Autodesk Inventor part; units mm, degrees
ref_plane "YZ Plane" through (0, 0, 0) normal (1, 0, 0) x (0, 1, 0)
ref_plane "XZ Plane" through (0, 0, 0) normal (0, 1, 0) x (-1, 0, 0)
ref_plane "XY Plane" through (0, 0, 0) normal (0, 0, 1) x (1, 0, 0)
sketch "Sketch1" plane through (0, 0, 0) normal (0, 1, 0) x (-1, 0, 0)
  line L0 (0, 0) -> (37, 0)
  line L1 (37, 0) -> (37, -119)
  line L2 (37, -119) -> (0, -119)
  line L3 (0, -119) -> (0, 0)
  dimension "d0" = 37
  dimension "d1" = 119
extrude "Extrusion1" add sketch "Sketch1" along normal blind 2
sketch "Sketch3" plane through (0, 0, 0) normal (0, -1, 0) x (1, 0, 0)
  line L0 (0, 0) -> (-16.5, 0)
  line L1 (-37, 0) -> (0, 0)
  line L2 (-19, 0) -> (-19, -2)
  arc A0 (-21.5, -2) -> (-16.5, -2) centre (-19, -2) ccw
  line L3 (0, 0) -> (0, -119)
  line L4 (0, -119) -> (-19, -119)
  line L5 (0, -119) -> (-37, -119)
  line L6 (-19, -119) -> (-19, -117)
  arc A1 (-16.5, -117) -> (-21.5, -117) centre (-19, -117) ccw
  line L7 (-16.5, -117) -> (-16.5, -119)
  line L8 (-21.5, -117) -> (-21.5, -119)
  line L9 (-21.5, -119) -> (-16.5, -119)
  line L10 (-21.5, -2) -> (-21.5, 0)
  line L11 (-16.5, -2) -> (-16.5, 0)
  line L12 (-21.5, 0) -> (-16.5, 0)
  dimension "d14" = 19
  dimension "d15" = 2
  dimension "d16" = 5
  dimension "d17" = 19
  dimension "d18" = 2
  dimension "d19" = 5
extrude "Extrusion3" cut sketch "Sketch3" against normal blind 2
sketch "Sketch4" plane through (0, 2, 0) normal (0, 1, 0) x (1, 0, 0)
  line L0 (0, 119) -> (0, 0)
  line L1 (0, 0) -> (0, 12)
  line L2 (0, 12) -> (-6, 12)
  line L3 (-32, 12) -> (-32, 105)
  line L4 (-6, 105) -> (-6, 12)
  line L5 (-11.7, 105) -> (-11.7, 108.4)
  line L6 (-11.7, 108.4) -> (-10.4, 108.4)
  line L7 (-10.4, 108.4) -> (-10.4, 105)
  line L8 (-6, 12) -> (-8, 12)
  line L9 (-8, 12) -> (-8, 105)
  line L10 (-11.7, 105) -> (-11.7, 102)
  line L11 (-11.7, 102) -> (-10.2, 102)
  line L12 (-10.2, 102) -> (-10.2, 15)
  line L13 (-32, 105) -> (-11.7, 105)
  line L14 (-10.2, 15) -> (-11.7, 15)
  line L15 (-11.7, 15) -> (-11.7, 12)
  line L16 (-11.7, 12) -> (-11.7, 8.6)
  line L17 (-11.7, 8.6) -> (-10.4, 8.6)
  line L18 (-10.4, 8.6) -> (-10.4, 12)
  line L19 (-10.4, 12) -> (-8, 12)
  line L20 (-6, 105) -> (-8, 105)
  line L21 (-8, 105) -> (-10.4, 105)
  line L22 (-32, 12) -> (-11.7, 12)
  point P0 (-19, 2)
  dimension "d59" = 12
  dimension "d60" = 6
  dimension "d61" = 26
  dimension "d62" = 93
  dimension "d73" = 2
  dimension "d121" = 2
  dimension "d122" = 93
  dimension "d125" = 20.3
  dimension "d126" = 20.3
  dimension "d127" = 3.4
  dimension "d128" = 3.4
  dimension "d129" = 87
  dimension "d130" = 2.2
  dimension "d154" = 1.3
  dimension "d155" = 1.3
  dimension "d156" = 4.4
  dimension "d157" = 4.4
  dimension "d158" = 1.5
  dimension "d159" = 1.5
extrude "Extrusion7" add sketch "Sketch4" against normal blind 92 contours L15 L14 L12 L11 L10 L5 L6 L7 L21 L9 L19 L18 L17 L16
sketch "Sketch6" plane through (-10.2, -90, -102) normal (-1, 0, 0) x (0, 0, 1)
  line L0 (102, 92) -> (-17, 92)
  line L1 (-6.4, 92) -> (58.6, 92)
  line L2 (58.6, 92) -> (58.6, 66.128)
  circle A0 centre (58.6, 66.128) radius 1.375
  line L3 (-6.4, 90) -> (-6.4, 0)
  line L4 (58.6, 66.128) -> (58.6, 8.128)
  circle A1 centre (58.6, 8.128) radius 1.375
  line L5 (58.6, 8.128) -> (9.6, 8.128)
  circle A2 centre (9.6, 8.128) radius 1.375
  line L6 (9.6, 8.128) -> (9.6, 66.128)
  circle A3 centre (9.6, 66.128) radius 1.375
  point P0 (102, 90)
  dimension "d80" = 65
  dimension "d81" = 25.872
  dimension "d82" = 2.75
  dimension "d83" = 65
  dimension "d87" = 58
  dimension "d88" = 2.75
  dimension "d89" = 49
  dimension "d90" = 2.75
  dimension "d91" = 2.75
extrude "Extrusion8" cut sketch "Sketch6" against normal blind 2.2
sketch "Sketch7" plane through (0, 0, 0) normal (0, -1, 0) x (1, 0, 0)
  line L0 (-10.2, -102) -> (-10.2, -15)
  line L1 (-10.2, -102) -> (-10.2, -40)
  line L2 (-10.2, -40) -> (-13.1, -40)
  line L3 (-13.1, -40) -> (-29.1, -40)
  line L4 (-29.1, -40) -> (-29.1, -94)
  line L5 (-29.1, -94) -> (-13.1, -94)
  line L6 (-13.1, -94) -> (-13.1, -40)
  point P0 (0, 0)
  point P1 (-10, -12)
  point P2 (-10.2, -15)
  dimension "d94" = 62
  dimension "d95" = 2.9
  dimension "d96" = 16
  dimension "d97" = 54
extrude "Extrusion9" cut sketch "Sketch7" against normal blind 2
sketch "Sketch9" plane through (0, 2, 0) normal (0, 1, 0) x (1, 0, 0)
  line L0 (0, 0) -> (0, 119)
  arc A0 (-16.5, 2) -> (-21.5, 2) centre (-19, 2) ccw
  line L1 (-19, 2) -> (-19, 8.5)
  line L2 (-37, 0) -> (-37, 119)
  line L3 (-37, 8.5) -> (-32, 8.5)
  line L4 (-32, 8.5) -> (-12, 8.5)
  line L5 (-12, 8.5) -> (-12, 12.5)
  line L6 (-12, 12.5) -> (-32, 12.5)
  line L7 (-32, 12.5) -> (-32, 8.5)
  line L8 (-37, 0) -> (-21.5, 0)
  arc A1 (-21.5, 117) -> (-16.5, 117) centre (-19, 117) ccw
  line L9 (-19, 117) -> (-19, 110.5)
  line L10 (-37, 110.5) -> (-32, 110.5)
  line L11 (-32, 110.5) -> (-12, 110.5)
  line L12 (-12, 110.5) -> (-12, 106.5)
  line L13 (-12, 106.5) -> (-32, 106.5)
  line L14 (-32, 106.5) -> (-32, 110.5)
  line L15 (-21.5, 119) -> (-37, 119)
  dimension "d142" = 6.5
  dimension "d143" = 5
  dimension "d144" = 20
  dimension "d145" = 4
  dimension "d146" = 12.5
  dimension "d147" = 6.5
  dimension "d148" = 5
  dimension "d149" = 20
  dimension "d150" = 4
  dimension "d151" = 12.5
extrude "Extrusion11" cut sketch "Sketch9" against normal blind 2
properties part number "Slot"
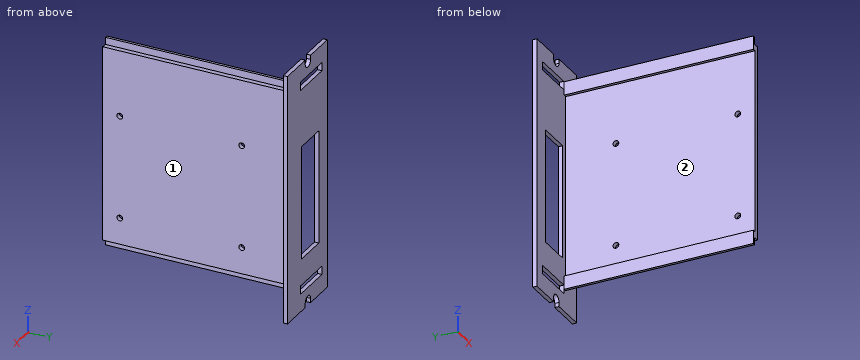
Check sheet for the modelled part. Datum: model origin and axes. Units: mm. Face numbers are marked on the shaded views. Give positions to 0.01 mm unless a question says otherwise; leave off trailing zeros. Order: outer loops, then holes, each group sorted by start corner. A loop starts at its lowest first (then second) coordinate and runs counter-clockwise, first axis right, second up. Notation, with made-up numbers: M 50.5,31.5 L 82.5,31.5 A32 ccw 82.5,65.5 Z; hole C -13,25.5 d11. An arc over 180 degrees is marked long. Answer in a Markdown table with one row per item. Add a question column.
Q1. Thickness scan on L1, parallel to Y at x = -9.1, z = -92.4; L2, parallel to X at y = -55.5, z = -24; L3, parallel to Y at x = -2, z = -11. Record the ranges inside material, lowest first.
Q2. Sectioned sample at A-A, the plane z = -75.5. Record the boundary of the cut face in (x, y).
Q3. Gauge pin test, flat ends, axial feed: pin 1 Ø7 at (y, z) = (-56, -11.5) entering from -X; pin 2 Ø0.6 at (x, y) = (-11, -41) entering from -Z; pin 3 Ø4.5 at (y, z) = (-81.872, -92.4) entering from -X. Record the tip position at first contact, or that the pin passes through.
Q4. Release check for a two-part mould opening along Z. For the marked faces 1 and 2 record: released by +Z, released by -Z, zero draft, split by the parting line, or undercut.
Q5. Sectioned sample at C-C, the plane z = -98.5. Record the boundary of the cut face in (x, y).
Q6. Sectioned sample at D-D, the plane y = -8. Record the boundary of the cut face in (x, z), and give its area (3 significant figures).
Q7. Sectioned sample at B-B, the plane x = -19. Record the boundary of the cut face in (y, z), and give its area (3 significant figures).
Verdict:
| question | item | result |
|---|---|---|
| 1 | L1 | -90 to -83.25, -80.5 to -25.25, -22.5 to 2 |
| 1 | L2 | -10.2 to -8 |
| 1 | L3 | 0 to 2 |
| 2 | outline | M -37,0 L -29.1,0 L -29.1,2 L -37,2 Z; M -13.1,0 L -10.2,0 L -10.2,-90 L -8,-90 L -8,0 L 0,0 L 0,2 L -13.1,2 Z |
| 3 | pin 1 | x = -11.7 |
| 3 | pin 2 | z = -108.4 |
| 3 | pin 3 | x = -10.2 |
| 4 | face 1 | zero draft |
| 4 | face 2 | undercut |
| 5 | outline | M -37,0 L -10.2,0 L -10.2,-90 L -8,-90 L -8,0 L 0,0 L 0,2 L -37,2 Z |
| 6 | outline | M -11.7,-108.4 L -10.4,-108.4 L -10.4,-105 L -8,-105 L -8,-12 L -10.4,-12 L -10.4,-8.6 L -11.7,-8.6 L -11.7,-15 L -10.2,-15 L -10.2,-102 L -11.7,-102 Z |
| 6 | area | 222 mm² |
| 7 | outline | M 0,-114.5 L 2,-114.5 L 2,-110.5 L 0,-110.5 Z; M 0,-106.5 L 2,-106.5 L 2,-94 L 0,-94 Z; M 0,-40 L 2,-40 L 2,-12.5 L 0,-12.5 Z; M 0,-8.5 L 2,-8.5 L 2,-4.5 L 0,-4.5 Z |
| 7 | area | 96.0 mm² |
